For this review, take the finished solid that the model builds, in its own axes (mm). Coordinates: 2 decimals unless noted, no trailing zeros. Order: outer loops, then holes, each group sorted by start corner. A loop starts at its lowest first (then second) coordinate and runs counter-clockwise, first axis right, second up. Notation, with made-up numbers: (21, 0) - (34, 0) arc R28 ccw to (34, 23) - close; hole circle Ø6 at (8, -17). An arc over 180 degrees is marked (long way). One line per item, written item: value. Start each with the question number.
(1) Consider section C-C on y = -1.15. Write out the cut boundary in (x, z) (3 decimals), then the cut area to 3 significant figures.
(2) Consider section B-B on z = 3. Write out the cut boundary in (x, y) (3 decimals).
(3) Mouldability with a two-part tool opening along X and no side actions: class faces 1 (the flat face through (9.5, -2, 8.1)), 2 (the cylindrical face through (20.626, -1.014, 3.06)), 3 (the flat face through (0, -1, 6)), 4 (the cylindrical face through (24.1, -1.01, 15.14)) as released by +X, released by -X, zero draft, split by the parting line, or undercut.
(4) Consider section D-D on z = 8. Write out the cut boundary in (x, y).
(5) Consider section A-A on x = 12.5. Write out the cut boundary in (y, z), then the cut area to 3 significant figures.
(6) To check wall thickness, follow line 1 along Z through (x, y) = (3, -1.2) (3 decimals); line 2 along Z through (x, y) = (12.5, -0.85); line 3 along Z through (x, y) = (3.5, -1.6). State the ranges of each line that lie inside material, in increasing order.
```python
from build123d import *

# Parameters (mm, degrees)
F0_W      = 25
F0_H      = 16
F1_DEPTH  = 2
F2_R      = 1.375
F6_DEPTH  = 3
F3_R      = 1.375
F7_DEPTH  = 3
F4_R      = 1.375
F8_DEPTH  = 3
F5_R      = 1.375
F9_DEPTH  = 3
F10_R     = 3
F11_R     = 3
F12_R     = 2.5
F13_DEPTH = 3


with BuildPart() as f1:
    # F0 (on Front) → F1 (new body)
    with BuildSketch(Plane.XZ):
        with Locations((12.5, 8)):
            Rectangle(F0_W, F0_H)
    extrude(amount=F1_DEPTH)

    # F2 (on face) → F6 (cut)
    with BuildSketch(Plane.XZ.offset(2)):
        with Locations((3, 13)):
            Circle(F2_R)
    extrude(amount=-F6_DEPTH, mode=Mode.SUBTRACT)

    # F3 (on face) → F7 (cut)
    with BuildSketch(Plane.XZ.offset(2)):
        with Locations((3, 3)):
            Circle(F3_R)
    extrude(amount=-F7_DEPTH, mode=Mode.SUBTRACT)

    # F4 (on face) → F8 (cut)
    with BuildSketch(Plane.XZ.offset(2)):
        with Locations((22, 13)):
            Circle(F4_R)
    extrude(amount=-F8_DEPTH, mode=Mode.SUBTRACT)

    # F5 (on face) → F9 (cut)
    with BuildSketch(Plane.XZ.offset(2)):
        with Locations((22, 3)):
            Circle(F5_R)
    extrude(amount=-F9_DEPTH, mode=Mode.SUBTRACT)

    # F10
    f10_edges = [f1.edges().sort_by_distance(p)[0] for p in [
        (25, -1, 16),
    ]]
    fillet(f10_edges, radius=F10_R)

    # F11
    f11_edges = [f1.edges().sort_by_distance(p)[0] for p in [
        (0, -1, 16),
    ]]
    fillet(f11_edges, radius=F11_R)

    # F12 (on face) → F13 (cut)
    with BuildSketch(Plane.XZ.offset(2)):
        with Locations((12.5, 8)):
            Circle(F12_R)
    extrude(amount=-F13_DEPTH, mode=Mode.SUBTRACT)


solid = f1.part
```
Geometry check:
1. outline: (0, 0) - (25, 0) - (25, 13) arc R3 ccw to (22, 16) - (3, 16) arc R3 ccw to (0, 13) - close; hole circle Ø2.75 at (3, 3); hole circle Ø2.75 at (3, 13); hole circle Ø5 at (12.5, 8); hole circle Ø2.75 at (22, 3); hole circle Ø2.75 at (22, 13)
1. area: 353 mm^2
2. outline: (0, -2) - (1.625, -2) - (1.625, 0) - (0, 0) - close; (4.375, -2) - (20.625, -2) - (20.625, 0) - (4.375, 0) - close; (23.375, -2) - (25, -2) - (25, 0) - (23.375, 0) - close
3. face 1: zero draft
3. face 2: undercut
3. face 3: released by -X
3. face 4: released by +X
4. outline: (0, -2) - (10, -2) - (10, 0) - (0, 0) - close; (15, -2) - (25, -2) - (25, 0) - (15, 0) - close
5. outline: (-2, 0) - (0, 0) - (0, 5.5) - (-2, 5.5) - close; (-2, 10.5) - (0, 10.5) - (0, 16) - (-2, 16) - close
5. area: 22.0 mm^2
6. line 1: z = 0 to 1.625, 4.375 to 11.625, 14.375 to 16
6. line 2: z = 0 to 5.5, 10.5 to 16
6. line 3: z = 0 to 1.72, 4.28 to 11.72, 14.28 to 16
